Autodesk Inventor part; units mm, degrees
ref_plane "YZ Plane" through (0, 0, 0) normal (1, 0, 0) x (0, 1, 0)
ref_plane "XZ Plane" through (0, 0, 0) normal (0, 1, 0) x (-1, 0, 0)
ref_plane "XY Plane" through (0, 0, 0) normal (0, 0, 1) x (1, 0, 0)
sketch "Sketch1" plane through (0, 0, 0) normal (0, 0, 1) x (1, 0, 0)
  circle A0 centre (0, 0) radius 47.625
  dimension "d0" = 95.25
extrude "Extrusion1" add sketch "Sketch1" along normal blind 3.175
sketch "Sketch3" plane through (0, 0, 3.175) normal (0, 0, 1) x (1, 0, 0)
  line L0 (1.27, 9.525) -> (20.32, 9.525)
  line L1 (20.32, 9.525) -> (20.32, 0)
  line L2 (20.32, 0) -> (1.27, 0)
  line L3 (1.27, 0) -> (1.27, 9.525)
  line L4 (0, 0) -> (0, -11.0035)
  line L5 (-1.27, 9.525) -> (-20.32, 9.525)
  line L6 (-20.32, 9.525) -> (-20.32, 0)
  line L7 (-20.32, 0) -> (-1.27, 0)
  line L8 (-1.27, 0) -> (-1.27, 9.525)
  dimension "d11" = 19.05
  dimension "d12" = 9.525
  dimension "d13" = 1.27
  dimension "d14" = 0
extrude "Extrusion3" add sketch "Sketch3" along normal blind 6.604
sketch "Sketch4" plane through (1.27, 9.525, 3.175) normal (0, 1, 0) x (1, 0, 0)
  circle A0 centre (4.445, -2.794) radius 1.27
  line L0 (19.05, -6.604) -> (0, -6.604)
  circle A1 centre (14.605, -2.794) radius 1.27
  line L1 (9.525, -6.604) -> (9.525, -7.9119)
  line L2 (-1.27, 3.175) -> (-1.27, 8.3959)
  circle A2 centre (-6.985, -2.794) radius 1.27
  circle A3 centre (-17.145, -2.794) radius 1.27
  dimension "d17" = 2.54
  dimension "d18" = 3.81
  dimension "d19" = 2.54
  dimension "d20" = 3.81
  dimension "d21" = 10.16
  dimension "d22" = 5.08
extrude "Extrusion4" cut sketch "Sketch4" against normal through all
sketch "Sketch5" plane through (0, 0, 3.175) normal (0, 0, 1) x (1, 0, 0)
  circle A0 centre (20.795, 25.8191) radius 3.175
  line L0 (0, 0) -> (0, 16.9345)
  circle A1 centre (-20.795, 25.8191) radius 3.175
  dimension "d25" = 6.35
  dimension "d26" = 20.795
  dimension "d27" = 25.8191
extrude "Extrusion5" cut sketch "Sketch5" against normal blind 25.4
sketch "Sketch6" plane through (0, 0, 3.175) normal (0, 0, 1) x (1, 0, 0)
  line L0 (0, 0) -> (0, 41.91)
  circle A0 centre (0, 41.91) radius 1.5875
  circle A1 centre (-36.2951, 20.955) radius 1.5875
  circle A2 centre (-36.2951, -20.955) radius 1.5875
  circle A3 centre (0, -41.91) radius 1.5875
  circle A4 centre (36.2951, -20.955) radius 1.5875
  circle A5 centre (36.2951, 20.955) radius 1.5875
  dimension "d30" = 41.91
  dimension "d31" = 3.175
  dimension "d34" = 360
extrude "Extrusion6" cut sketch "Sketch6" against normal blind 25.4
sketch "Sketch7" plane through (0, 0, 3.175) normal (0, 0, 1) x (1, 0, 0)
  line L0 (-28.575, -20.3352) -> (-20.32, -20.3352)
  line L1 (-20.32, -20.3352) -> (-20.32, -43.0725)
  line L2 (-28.575, -38.1) -> (-28.575, -20.3352)
  circle A0 centre (-24.13, -24.6888) radius 1.27
  circle A1 centre (-24.13, -34.8488) radius 1.27
  circle A2 centre (0, 0) radius 47.625
  line L3 (0, 0) -> (0, -12.4863)
  line L4 (28.575, -20.3352) -> (20.32, -20.3352)
  line L5 (20.32, -20.3352) -> (20.32, -43.0725)
  line L6 (28.575, -38.1) -> (28.575, -20.3352)
  circle A3 centre (24.13, -24.6888) radius 1.27
  circle A4 centre (24.13, -34.8488) radius 1.27
  arc A5 (20.32, -43.0725) -> (28.575, -38.1) centre (0, 0) ccw
  dimension "d38" = 20.32
  dimension "d39" = 2.54
  dimension "d40" = 2.54
  dimension "d41" = 24.6888
  dimension "d42" = 10.16
  dimension "d43" = 3.81
  dimension "d44" = 8.255
extrude "Extrusion7" add sketch "Sketch7" along normal blind 31.75 contours L0 L1 A2 L2 | L5 L4 L6 A2
sketch "Sketch8" plane through (0, 0, 34.925) normal (0, 0, 1) x (1, 0, 0)
  circle A0 centre (24.13, -24.6888) radius 1.27
  circle A1 centre (24.13, -34.8488) radius 1.27
  line L0 (20.32, -20.3352) -> (20.32, -43.0725)
  line L1 (20.32, -43.0725) -> (20.32, -20.3352)
  line L2 (24.13, -31.2293) -> (20.32, -31.2293)
  line L3 (20.32, -31.2293) -> (20.32, -28.0543)
  line L4 (20.32, -28.0543) -> (24.13, -28.0543)
  line L5 (24.13, -28.0543) -> (24.13, -31.2293)
  point P0 (0, 0)
  dimension "d47" = 3.175
  dimension "d48" = 3.3655
extrude "Extrusion8" cut sketch "Sketch8" against normal up to surface (31.75 mm away) contours L4 L5 L2 L0
fillet "Fillet1" radius 3.175 2 edges at (20.32, -28.0543, 19.05) (20.32, -31.2293, 19.05)
properties part number "rearServoAttachmentPlate" material "ABS Plastic"
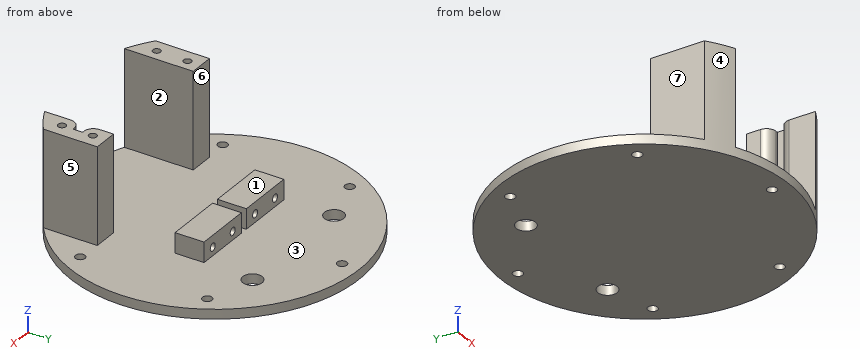
Could you check a few things on this model? Use its own coordinates, in mm. Face numbers are marked on the shaded views. A direction names the side the tool comes from. Give positions to 0.01 mm unless a question says otherwise; leave off trailing zeros. Order: outer loops, then holes, each group sorted by start corner. A loop starts at its lowest first (then second) coordinate and runs counter-clockwise, first axis right, second up.
1. For the marked faces 5, 6 and 7, which set-ups out of +Z, -Z, +X, -X, +Y, -Y let a thin tool reach every point of the face, with its end or its side?
2. Suppose I cut it at A-A (x = 0). List the corners of the cut face in (y, z) for me (1 decimal).
3. Suppose I cut it at B-B (y = -41.91). List the corners of the cut face in (x, z) for me (1 decimal).
4. I need wall thicknesses on L1, parallel to Y at x = 24, z = 15; L2, parallel to X at y = -22, z = 29.5 (3 decimals); L3, parallel to Z at x = -39, y = 15 (3 decimals). Which ranges of each line are inside material? Lowest first, please.
5. We'd pull the mould along X, two halves only. Please class the marked faces 1, 2, 3 and 4: pulls with the +X half, pulls with the -X half, needs draft (parallel to the pull), parting line crosses it, or undercut.
6. Suppose I cut it at D-D (y = 7.5). List the corners of the cut face in (x, z) for me (3 decimals).
7. Suppose I cut it at C-C (z = 12). Give the number of separate pieces and of enclosed holes in the cut face, plus the area to 3 significant figures.
8. Will these pins go through, and if not, where does the flat tip stop? P1, Ø10, axis at y = 28.5, z = 4, coming from the -X side; P2, Ø0.8, axis at x = 24, y = -25, coming from the +Z side (3 decimals); P3, Ø3.5, axis at y = 6, z = 5, coming from the +X side.
Solved:
1. face 5: +Z, +X, +Y, -Y
1. face 6: +Z, +X, -X, +Y
1. face 7: +Z, -X, +Y, -Y
2. outline: (-47.6, 0) - (-43.5, 0) - (-43.5, 3.2) - (-47.6, 3.2) - close; (-40.3, 0) - (40.3, 0) - (40.3, 3.2) - (-40.3, 3.2) - close; (43.5, 0) - (47.6, 0) - (47.6, 3.2) - (43.5, 3.2) - close
3. outline: (-22.6, 0) - (-1.6, 0) - (-1.6, 3.2) - (-20.3, 3.2) - (-20.3, 34.9) - (-22.6, 34.9) - close; (1.6, 0) - (22.6, 0) - (22.6, 34.9) - (20.3, 34.9) - (20.3, 3.2) - (1.6, 3.2) - close
4. L1: y = -41.14 to -36.11, -33.59 to -31.23, -28.05 to -25.95, -23.43 to -20.34
4. L2: x = -28.575 to -20.32, 20.32 to 28.575
4. L3: z = 0 to 3.175
5. face 1: needs draft
5. face 2: undercut
5. face 3: undercut
5. face 4: parting line crosses it
6. outline: (-47.031, 0) - (47.031, 0) - (47.031, 3.175) - (20.32, 3.175) - (20.32, 9.779) - (1.27, 9.779) - (1.27, 3.175) - (-1.27, 3.175) - (-1.27, 9.779) - (-20.32, 9.779) - (-20.32, 3.175) - (-47.031, 3.175) - close; hole circle Ø2.54 at (-15.875, 5.969); hole circle Ø2.54 at (-5.715, 5.969); hole circle Ø2.54 at (5.715, 5.969); hole circle Ø2.54 at (15.875, 5.969)
7. separate pieces: 2
7. enclosed holes: 4
7. area: 301 mm2
8. P1: stops at x = -41.38
8. P2: stops at z = 3.175
8. P3: stops at x = 20.32
